```python
from build123d import *

# Parameters (mm, degrees)
SKETCH_W        = 42
SKETCH_H        = 42
PAD_DEPTH       = 47
SKETCH001_R     = 1.5
POCKET_DEPTH    = 5
POCKET001_DEPTH = 47
SKETCH003_R     = 16
POCKET002_DEPTH = 1
SKETCH004_R     = 11
PAD001_DEPTH    = 2
SKETCH005_R     = 2.5
PAD002_DEPTH    = 22
SKETCH006_W     = 8
SKETCH006_H     = 7
PAD003_DEPTH    = 1


with BuildPart() as part:
    # Sketch → Pad (new body)
    with BuildSketch(Plane.YZ):
        Rectangle(SKETCH_W, SKETCH_H)
    extrude(amount=PAD_DEPTH)

    # Sketch001 → Pocket (cut)
    with BuildSketch(Plane.YZ.offset(47)):
        with Locations((15.5, 15.5)):
            Circle(SKETCH001_R)
        with Locations((-15.5, 15.5)):
            Circle(SKETCH001_R)
        with Locations((-15.5, -15.5)):
            Circle(SKETCH001_R)
        with Locations((15.5, -15.5)):
            Circle(SKETCH001_R)
    extrude(amount=-POCKET_DEPTH, mode=Mode.SUBTRACT)

    # Sketch002 → Pocket001 (cut)
    with BuildSketch(Plane.YZ.offset(47)):
        Polygon((-21, 21), (-21, 17.183766), (-17.183766, 21), align=None)
        Polygon((21, 21), (17.183766, 21), (21, 17.183766), align=None)
        Polygon((21, -21), (21, -17.183766), (17.183766, -21), align=None)
        Polygon((-21, -21), (-21, -17.183766), (-17.183766, -21), align=None)
    extrude(amount=-POCKET001_DEPTH, mode=Mode.SUBTRACT)

    # Sketch003 → Pocket002 (cut)
    with BuildSketch(Plane.YZ.offset(47)):
        Circle(SKETCH003_R)
    extrude(amount=-POCKET002_DEPTH, mode=Mode.SUBTRACT)

    # Sketch004 → Pad001 (new body)
    with BuildSketch(Plane.YZ.offset(46)):
        Circle(SKETCH004_R)
    extrude(amount=PAD001_DEPTH)

    # Sketch005 → Pad002 (new body)
    with BuildSketch(Plane.YZ.offset(48)):
        Circle(SKETCH005_R)
    extrude(amount=PAD002_DEPTH)

    # Sketch006 → Pad003 (new body)
    with BuildSketch(Plane(origin=(0, 0, 21), x_dir=(0, -1, 0), z_dir=(0, 0, 1))):
        with Locations((0, 5)):
            Rectangle(SKETCH006_W, SKETCH006_H)
    extrude(amount=PAD003_DEPTH)


solid = part.part
```
The model under review builds one solid part; all positions refer to its coordinate system, in mm. A direction names the side the tool comes from. Coordinates: 2 decimals unless noted, no trailing zeros. Write each loop counter-clockwise with the first axis right and the second up, starting at its lowest first coordinate (ties: lowest second). Pieces come first, ordered by that corner, then holes.
1) To check wall thickness, follow probe 1 along Z at (x, y) = (45, -15.5); probe 2 along Z at (x, y) = (46.8, 0); probe 3 along Y at (x, z) = (45, -15). State the ranges of each line that lie inside material, in increasing order.
2) We need section C-C on z = 0. State the section outline as (x, y) points.
3) Clearance check with flat-ended pins moving along their axes: pin 1 Ø3 at (x, z) = (54, 5) entering from -Y; pin 2 Ø2.5 at (y, z) = (-15.5, -15.5) entering from -X; pin 3 Ø1.1 at (x, z) = (4, 21.5) entering from -Y; pin 4 Ø3.5 at (y, z) = (15.5, -15) entering from +X. State where each tip first meets the part, or that it passes through.
4) Machinability: for faces 1 (the face through (23, 0, -21)), 2 (the face through (42, 15, -15)), which of the approach directions +Z, -Z, +X, -X, +Y, -Y give a long, thin tool a straight path to every point of the face, cutting with its end or side? Answer none if there is none.
5) We need section D-D on x = 59. State the section outline as (y, z) points.
6) We need section B-B on y = 0. State the section outline as (x, z) points.
7) We need section A-A on x = 6.5. State the section outline as (y, z) points.
8) The part is to be moulded in two halves that separate along Z. For faces 3 (the face through (44.54, -17, 15.57)), 4 (the face through (70, 0, 0)), 5 (the face through (23.829, 19.065, 19.119)), say which applies: pulls with the +Z half, pulls with the -Z half, needs draft (parallel to the pull), parting line crosses it, or undercut.
Answer list:
1. probe 1: z = -21 to -17, -14 to 14, 17 to 21
1. probe 2: z = -21 to -16, -11 to 11, 16 to 21
1. probe 3: y = -21 to -16.91, -14.09 to 14.09, 16.91 to 21
2. outline: (0, -21) - (47, -21) - (47, -16) - (46, -16) - (46, -11) - (48, -11) - (48, -2.5) - (70, -2.5) - (70, 2.5) - (48, 2.5) - (48, 11) - (46, 11) - (46, 16) - (47, 16) - (47, 21) - (0, 21) - close
3. pin 1: passes through
3. pin 2: stops at x = 0
3. pin 3: stops at y = -17.23
3. pin 4: stops at x = 47
4. face 1: -Z, +X, -X, +Y, -Y
4. face 2: +X
5. outline: circle Ø5 at (0, 0)
6. outline: (0, -21) - (47, -21) - (47, -16) - (46, -16) - (46, -11) - (48, -11) - (48, -2.5) - (70, -2.5) - (70, 2.5) - (48, 2.5) - (48, 11) - (46, 11) - (46, 16) - (47, 16) - (47, 21) - (8.5, 21) - (8.5, 22) - (1.5, 22) - (1.5, 21) - (0, 21) - close
7. outline: (-21, -17.18) - (-17.18, -21) - (17.18, -21) - (21, -17.18) - (21, 17.18) - (17.18, 21) - (4, 21) - (4, 22) - (-4, 22) - (-4, 21) - (-17.18, 21) - (-21, 17.18) - close
8. face 3: undercut
8. face 4: needs draft
8. face 5: pulls with the +Z half
